Read the model definition and answer for the solid it produces. Units are mm, in the model's axes. Face numbers are marked on the shaded views. A direction names the side the tool comes from. Coordinates: 2 decimals unless noted, no trailing zeros. Loops run counter-clockwise (first coordinate to the right, second up) from the corner with the lowest first, then second, coordinate; pieces in that order, holes last.
from build123d import *

# Parameters (mm, degrees)
PAD019_DEPTH     = 18.5
POCKET042_DEPTH  = 13
POCKET043_DEPTH  = 5
POCKET044_DEPTH  = 15
CHAMFER018_SIZE  = 3
CHAMFER019_SIZE  = 2
CHAMFER020_SIZE  = 1
CHAMFER021_SIZE  = 1
CHAMFER022_SIZE  = 1
CHAMFER023_SIZE  = 1
CHAMFER024_SIZE  = 1
CHAMFER025_SIZE  = 1.5
CHAMFER026_SIZE  = 1
CHAMFER027_SIZE  = 1
CHAMFER028_SIZE  = 1
CHAMFER029_SIZE  = 1
CHAMFER030_SIZE  = 1.5
CHAMFER031_SIZE2 = 3
CHAMFER031_SIZE  = 10
CHAMFER032_SIZE2 = 10
CHAMFER032_SIZE  = 3
CHAMFER033_SIZE  = 1
CHAMFER034_SIZE  = 1.5
CHAMFER035_SIZE  = 1
SKETCH082_R      = 2.75
POCKET045_DEPTH  = 12
SKETCH083_R      = 1.7
POCKET046_DEPTH  = 5


with BuildPart() as part:
    # Sketch078 → Pad019 (new body)
    with BuildSketch(Plane.XY):
        Polygon((0, 38.8), (8, 38.8), (8, 40.6), (14, 40.6), (14, 38.8), (28, 38.8), (28, 40.6), (34, 40.6), (34, 38.7761214391), (37.3, 38.7761214391), (41.9953022309, 33.1864759261), (38.7027713123, 30.4207499545), (37.673663974, 31.6458777382), (31.9308774881, 26.82193709), (30.0013012288, 29.1190516844), (9.0209879336, 11.4955885164), (10.9505641929, 9.198473922), (0, 0), align=None)
        Polygon((7.5, 32.8), (7.5, 18.1), (25, 32.8), align=None, mode=Mode.SUBTRACT)
    extrude(amount=PAD019_DEPTH)

    # Sketch079 → Pocket042 (cut)
    with BuildSketch(Plane.XY.offset(6.5)):
        Polygon((0, 5.5542995553), (8.2661306752, 12.395656), (10.9598026716, 9.1854627211), (31.9879670751, 26.8301877163), (29.8577953381, 29.3688275367), (38.9152591587, 36.9689420879), (34.890976, 41.764896), (21, 41.764896), (21, 32.458794), (1, 32.458794), (1, 41.759258), (0, 41.764896), align=None)
    extrude(amount=POCKET042_DEPTH, mode=Mode.SUBTRACT)

    # Sketch080 → Pocket043 (cut)
    with BuildSketch(Plane.XY.offset(16.5)):
        Polygon((-0.8541061726, -4.3526620467), (49.194970654, 37.6434998606), (44.0526697777, 43.7718554052), (-5.9964070501, 1.7756934982), align=None)
    extrude(amount=POCKET043_DEPTH, mode=Mode.SUBTRACT)

    # Sketch081 → Pocket044 (cut)
    with BuildSketch(Plane.XY.offset(5.8)):
        Polygon((37.0972154509, 31.1536445146), (41.470166846, 34.8229864174), (44.3478623025, 31.3934825187), (39.9749109074, 27.724140616), align=None)
        Polygon((6.1, 34.25), (16.1, 34.25), (16.9452365235, 32.4373844259), (5.2547634765, 32.4373844259), align=None)
    extrude(amount=POCKET044_DEPTH, mode=Mode.SUBTRACT)

    # Chamfer018
    chamfer018_edges = [part.edges().sort_by_distance(p)[0] for p in [
        (39.915045, 35.662973, 16.5),
    ]]
    chamfer(chamfer018_edges, length=CHAMFER018_SIZE)

    # Chamfer019
    chamfer019_edges = [part.edges().sort_by_distance(p)[0] for p in [
        (5.475282, 4.599237, 0),
        (19.511145, 20.30732, 0),
        (34.802271, 29.233907, 0),
    ]]
    chamfer(chamfer019_edges, length=CHAMFER019_SIZE)

    # Chamfer020
    chamfer020_edges = [part.edges().sort_by_distance(p)[0] for p in [
        (9.342584, 11.112736, 0),
        (8.377796, 12.261293, 0),
        (29.358109, 29.884757, 0),
        (30.322897, 28.736199, 0),
    ]]
    chamfer(chamfer020_edges, length=CHAMFER020_SIZE)

    # Chamfer021
    chamfer021_edges = [part.edges().sort_by_distance(p)[0] for p in [
        (7.5, 25.45, 0),
        (16.25, 25.45, 0),
        (16.25, 32.8, 0),
    ]]
    chamfer(chamfer021_edges, length=CHAMFER021_SIZE)

    # Chamfer022
    chamfer022_edges = [part.edges().sort_by_distance(p)[0] for p in [
        (0, 20.705986, 0),
        (0, 22.17715, 6.5),
    ]]
    chamfer(chamfer022_edges, length=CHAMFER022_SIZE)

    # Chamfer023
    chamfer023_edges = [part.edges().sort_by_distance(p)[0] for p in [
        (0, 38.8, 3.25),
    ]]
    chamfer(chamfer023_edges, length=CHAMFER023_SIZE)

    # Chamfer024
    chamfer024_edges = [part.edges().sort_by_distance(p)[0] for p in [
        (0, 0, 9.25),
    ]]
    chamfer(chamfer024_edges, length=CHAMFER024_SIZE)

    # Chamfer025
    chamfer025_edges = [part.edges().sort_by_distance(p)[0] for p in [
        (0, 3.27715, 16.5),
    ]]
    chamfer(chamfer025_edges, length=CHAMFER025_SIZE)

    # Chamfer026
    chamfer026_edges = [part.edges().sort_by_distance(p)[0] for p in [
        (4.883065, 9.595706, 16.5),
    ]]
    chamfer(chamfer026_edges, length=CHAMFER026_SIZE)

    # Chamfer027
    chamfer027_edges = [part.edges().sort_by_distance(p)[0] for p in [
        (1.132852, 0.951596, 16.132852),
    ]]
    chamfer(chamfer027_edges, length=CHAMFER027_SIZE)

    # Chamfer028
    chamfer028_edges = [part.edges().sort_by_distance(p)[0] for p in [
        (8.266131, 12.395656, 11),
    ]]
    chamfer(chamfer028_edges, length=CHAMFER028_SIZE)

    # Chamfer029
    chamfer029_edges = [part.edges().sort_by_distance(p)[0] for p in [
        (38.079114, 37.848605, 6.5),
    ]]
    chamfer(chamfer029_edges, length=CHAMFER029_SIZE)

    # Chamfer030
    chamfer030_edges = [part.edges().sort_by_distance(p)[0] for p in [
        (31, 40.6, 6.5),
    ]]
    chamfer(chamfer030_edges, length=CHAMFER030_SIZE)

    # Chamfer031
    chamfer031_edges = [part.edges().sort_by_distance(p)[0] for p in [
        (21, 35.8, 18.5),
    ]]
    chamfer031_side = part.faces().sort_by_distance((21, 35.8, 12.5))[0]
    chamfer(chamfer031_edges, length=CHAMFER031_SIZE, length2=CHAMFER031_SIZE2, reference=chamfer031_side)

    # Chamfer032
    chamfer032_edges = [part.edges().sort_by_distance(p)[0] for p in [
        (1, 35.629397, 18.5),
    ]]
    chamfer032_side = part.faces().sort_by_distance((9.318343, 36.537604, 18.5))[0]
    chamfer(chamfer032_edges, length=CHAMFER032_SIZE, length2=CHAMFER032_SIZE2, reference=chamfer032_side)

    # Chamfer033
    chamfer033_edges = [part.edges().sort_by_distance(p)[0] for p in [
        (17.388073, 32.8, 18.5),
        (4.632373, 32.458794, 18.5),
    ]]
    chamfer(chamfer033_edges, length=CHAMFER033_SIZE)

    # Chamfer034
    chamfer034_edges = [part.edges().sort_by_distance(p)[0] for p in [
        (11, 40.6, 18.5),
    ]]
    chamfer(chamfer034_edges, length=CHAMFER034_SIZE)

    # Chamfer035
    chamfer035_edges = [part.edges().sort_by_distance(p)[0] for p in [
        (23, 32.8, 6.5),
        (16.25, 25.45, 6.5),
        (7.5, 25.268692, 6.5),
    ]]
    chamfer(chamfer035_edges, length=CHAMFER035_SIZE)

    # Sketch082 → Pocket045 (cut)
    with BuildSketch(Plane.XZ.offset(-30)):
        with Locations((11.1, 12.9)):
            Circle(SKETCH082_R)
    extrude(amount=-POCKET045_DEPTH, mode=Mode.SUBTRACT)

    # Sketch083 (on DatumPlane) → Pocket046 (cut)
    with BuildSketch(Plane(origin=(0, 0, 0), x_dir=(0.7657048648, 0.6431920864, 0), z_dir=(0.6431920864, -0.7657048648, 0))):
        with Locations((5, 10.6)):
            Circle(SKETCH083_R)
        with Locations((46, 10.6)):
            Circle(SKETCH083_R)
    extrude(amount=-POCKET046_DEPTH, mode=Mode.SUBTRACT)


with BuildPart() as part_1:
    # Body015 placement: moved
    add(part.part.moved(Location((57, 0, 0))))


solid = part_1.part
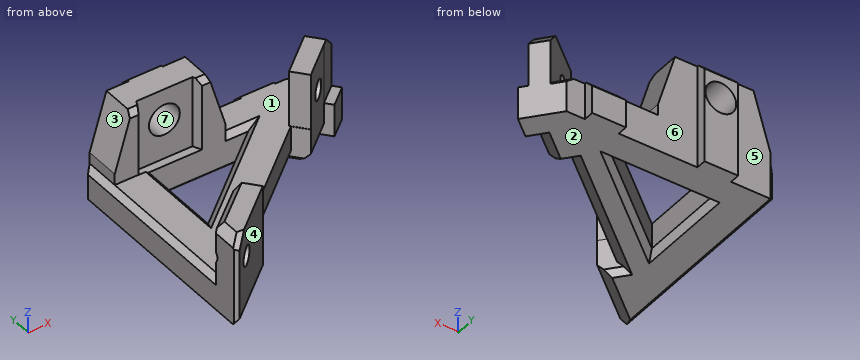
Item 1: A cutting plane is placed at C-C on y = 24.5. Determine the outline of the cut face in (x, z).
Numbers:
outline: (57, 1) - (58, 0) - (63.5, 0) - (64.5, 1) - (64.5, 5.5) - (63.5, 6.5) - (58, 6.5) - (57, 5.5) - close; (72.12, 1) - (73.67, 0) - (78.39, 0) - (81.5, 2) - (81.5, 6.5) - (73.67, 6.5) - (72.12, 5.5) - close
Item 2: Given pin 1 (8 mm diameter, centred on x = 69.5, z = 9.5, fed in from -Y); pin 2 (0.9 mm diameter, centred on y = 40, z = 2.5, fed in from +X); pin 3 (2.5 mm diameter, centred on y = 27, z = 4.5, fed in from +X); pin 4 (1.5 mm diameter, centred on y = 21.5, z = 9, fed in from +X), each flat-ended and moving along its own axis, determine where each tip first touches the part or whether it passes through.
Numbers:
pin 1: stops at y = 7.14
pin 2: stops at x = 91
pin 3: stops at x = 90.63
pin 4: passes through
Item 3: A cutting plane is placed at A-A on z = 12.9. Give the number of separate pieces and of enclosed holes in the cut face, then the cut area to 3 significant figures.
Numbers:
separate pieces: 4
enclosed holes: 0
area: 156 mm2
Item 4: A cutting plane is placed at D-D on y = 13. Determine the outline of the cut face in (x, z).
Numbers:
outline: (57, 1) - (58, 0) - (64.7, 0) - (67.81, 2) - (67.81, 6.5) - (58, 6.5) - (57, 5.5) - close
Item 5: Find the intervals of material crossed by line 1 along Z through (x, y) = (68.1, 38.75); line 2 along X through (y, z) = (36.5, 12); line 3 along Z through (x, y) = (59, 20), in increasing order.
Numbers:
line 1: z = 0 to 10.15, 15.65 to 18.5
line 2: x = 59.05 to 65.5, 70.7 to 76.95, 95.36 to 96.21
line 3: z = 0 to 6.5
Item 6: Determine the mould class of the marked faces 1, 2, 3 and 4 for opening direction X: released by +X, released by -X, zero draft, split by the parting line, or undercut.
Numbers:
face 1: undercut
face 2: zero draft
face 3: released by -X
face 4: released by +X
Item 7: A cutting plane is placed at B-B on z = 2.75. Determine the outline of the cut face in (x, y).
Numbers:
outline: (57, 1) - (57.77, 0.64) - (67.95, 9.2) - (66.02, 11.5) - (87, 29.12) - (88.93, 26.82) - (94.67, 31.65) - (95.7, 30.42) - (99, 33.19) - (94.3, 38.78) - (91, 38.78) - (91, 40.6) - (85, 40.6) - (85, 38.8) - (71, 38.8) - (71, 40.6) - (65, 40.6) - (65, 38.8) - (58, 38.8) - (57, 37.8) - close; hole (64.5, 18.1) - (82, 32.8) - (64.5, 32.8) - close
Item 8: Which of the six approach directions +Z, -Z, +X, -X, +Y, -Y give full straight-line access (tool end or side, diameter ignored) to the marked faces 5, 6 and 7?
Numbers:
face 5: +Z, -Z, -X, +Y
face 6: +Z, -Z, +Y
face 7: +Y
